Could you check a few things on this drawing? It's one solid part, dimensions in mm from its lowest x, y, z. Coordinates: 2 decimals unless noted, no trailing zeros. Write each loop counter-clockwise with the first axis right and the second up, starting at its lowest first coordinate (ties: lowest second). Pieces come first, ordered by that corner, then holes. Notation, with made-up numbers: (49.5, 1.5) - (104.5, 1.5) arc R9 cw to (104.5, 5.5) - close; hole circle Ø8 at (-38.75, 22.5). An arc over 180 degrees is marked (long way). Use one line per item in the form item = value. Start each with the question number.
(1) If we section it at A-A on x = 258.5: Please give me the cut outline in (y, z).
(2) If we section it at B-B on z = 104.5: Please give me the cut outline in (x, y).
(3) If I drill on probe 1 along Z at (x, y) = (133, 12.5); probe 2 along Y at (x, z) = (268, 246); probe 3 along X at (y, z) = (6.75, 149) (1 decimal), over which ranges is the centre line in solid material (lowest first)? Write a range as from..to.
(4) For pin 1 Ø2 at (x, y) = (73.5, 2) entering from -Z; pin 2 Ø7.5 at (x, z) = (107.5, 241) entering from +Y; pin 3 Ø5 at (y, z) = (5, 193.5) entering from -X (1 decimal); pin 4 Ø2 at (y, z) = (2.5, 215.5) entering from +X, each with a flat end and sliding along its axis, tell me the tip position at first contact or that it passes through.
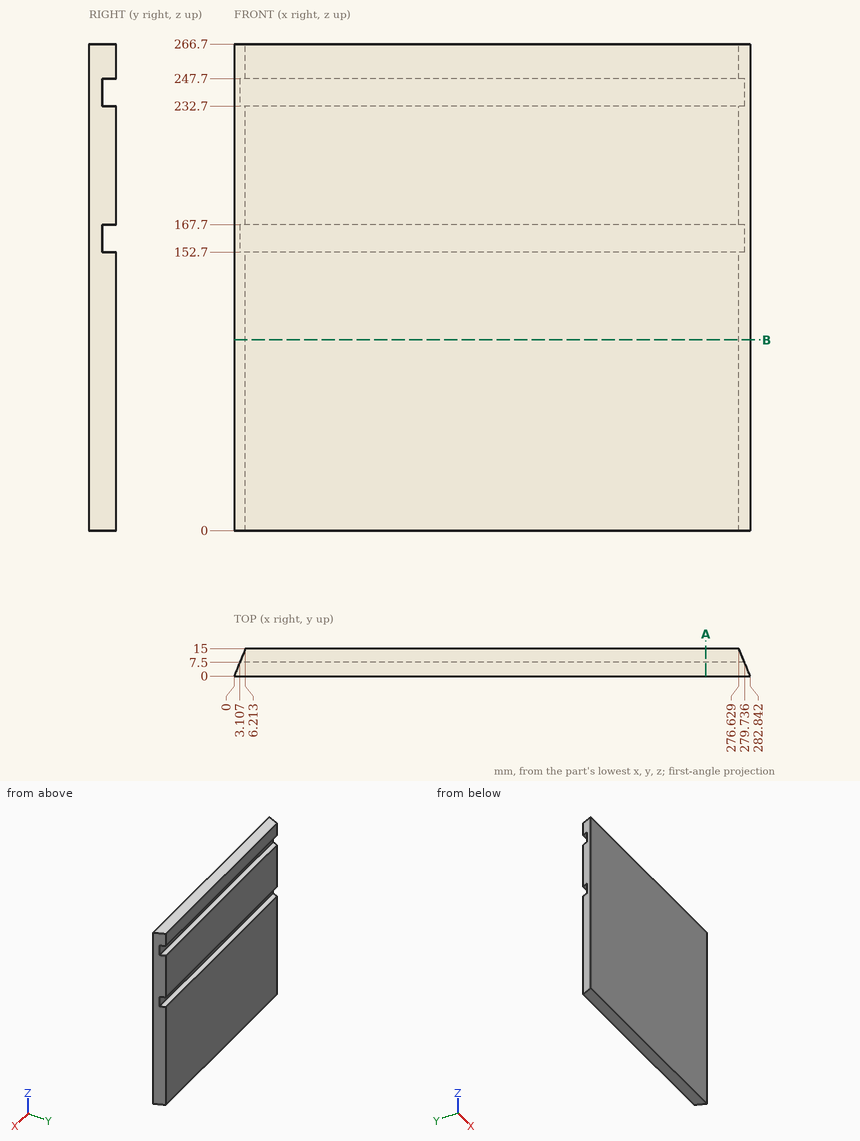
Reported:
q1.outline = (0, 0) - (15, 0) - (15, 152.7) - (7.5, 152.7) - (7.5, 167.7) - (15, 167.7) - (15, 232.7) - (7.5, 232.7) - (7.5, 247.7) - (15, 247.7) - (15, 266.7) - (0, 266.7) - close
q2.outline = (0, 0) - (282.84, 0) - (276.63, 15) - (6.21, 15) - close
q3.probe_1 = 0..152.7, 167.7..232.7, 247.7..266.7
q3.probe_2 = 0..7.5
q3.probe_3 = 2.8..280
q4.pin_1 = 0
q4.pin_2 = 7.5
q4.pin_3 = 1
q4.pin_4 = 282.22
